For this review, use the dimensioned drawing (mm, ordinates from the lowest corner) and the shaded views. Coordinates: 2 decimals unless noted, no trailing zeros. Loops run counter-clockwise (first coordinate to the right, second up) from the corner with the lowest first, then second, coordinate; pieces in that order, holes last.
1. Take a section at A-A, the plane y = 24. State the section outline as (x, z) points.
2. Take a section at B-B, the plane x = 4.25. State the section outline as (y, z) points.
3. To check wall thickness, follow probe 1 along Y at (x, z) = (4.25, 7); probe 2 along X at (y, z) = (24, 8.75); probe 3 along Y at (x, z) = (4.25, 3). State the ranges of each line that lie inside material, in increasing order.
4. Take a section at D-D, the plane y = 13.5. State the section outline as (x, z) points.
5. Mouldability with a two-part tool opening along X and no side actions: class the marked faces 1, 2, 3 and 4 as pulls with the +X half, pulls with the -X half, needs draft (parallel to the pull), parting line crosses it, or undercut.
6. Take a section at C-C, the plane z = 4.75. State the section outline as (x, y) points, then the cut area to 3 significant figures.
7. Clearance check with flat-ended pins moving along their axes: P1, Ø4, axis at y = 10, z = 3, coming from the +X side; P2, Ø2, axis at y = 9.5, z = 8.5, coming from the -X side; P3, Ø6.5, axis at y = 17, z = 3, coming from the -X side; P4, Ø1, axis at x = 7, y = 10.5, coming from the -Z side. State where each tip first meets the part, or that it passes through.
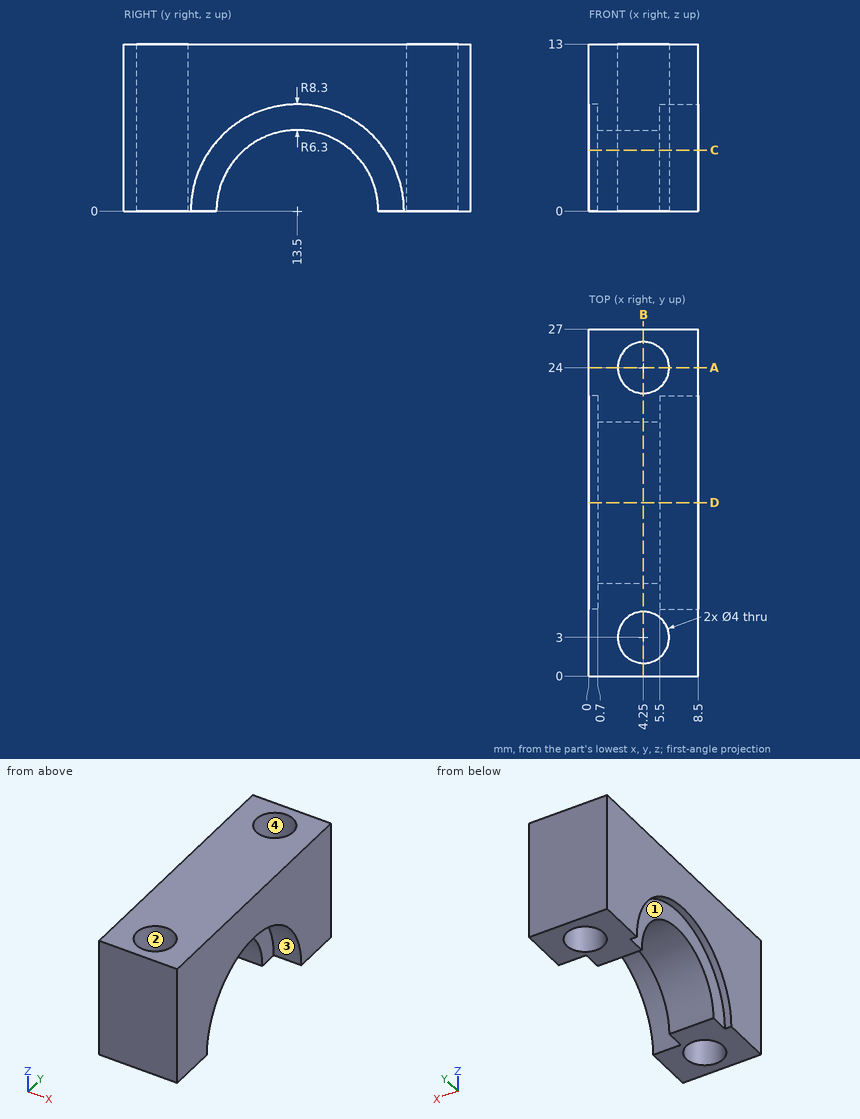
Results list:
1. outline: (0, 0) - (2.25, 0) - (2.25, 13) - (0, 13) - close; (6.25, 0) - (8.5, 0) - (8.5, 13) - (6.25, 13) - close
2. outline: (0, 0) - (1, 0) - (1, 13) - (0, 13) - close; (5, 0) - (7.2, 0) arc R6.3 cw to (19.8, 0) - (22, 0) - (22, 13) - (5, 13) - close; (26, 0) - (27, 0) - (27, 13) - (26, 13) - close
3. probe 1: y = 0 to 1, 5 to 22, 26 to 27
3. probe 2: x = 0 to 2.25, 6.25 to 8.5
3. probe 3: y = 0 to 1, 5 to 7.96, 19.04 to 22, 26 to 27
4. outline: (0, 8.3) - (0.7, 8.3) - (0.7, 6.3) - (5.5, 6.3) - (5.5, 8.3) - (8.5, 8.3) - (8.5, 13) - (0, 13) - close
5. face 1: pulls with the -X half
5. face 2: undercut
5. face 3: needs draft
5. face 4: undercut
6. outline: (0, 0) - (8.5, 0) - (8.5, 6.69) - (5.5, 6.69) - (5.5, 9.36) - (0.7, 9.36) - (0.7, 6.69) - (0, 6.69) - close; (0, 20.31) - (0.7, 20.31) - (0.7, 17.64) - (5.5, 17.64) - (5.5, 20.31) - (8.5, 20.31) - (8.5, 27) - (0, 27) - close; hole circle Ø4 at (4.25, 3); hole circle Ø4 at (4.25, 24)
6. area: 114 mm2
7. P1: stops at x = 5.5
7. P2: stops at x = 0
7. P3: stops at x = 0.7
7. P4: stops at z = 7.53
